Build history of the part. All positions in model axes, mm. Face numbers are marked on the shaded views. A direction names the side the tool comes from. Coordinates: 2 decimals unless noted, no trailing zeros. Order: outer loops, then holes, each group sorted by start corner. A loop starts at its lowest first (then second) coordinate and runs counter-clockwise, first axis right, second up. Notation, with made-up numbers: (-23, -3) - (26, -3) arc R19 cw to (26, 16) - close; hole circle Ø1 at (-28, 7). An arc over 180 degrees is marked (long way). Write each question's results on one line, items separated by ' | '.
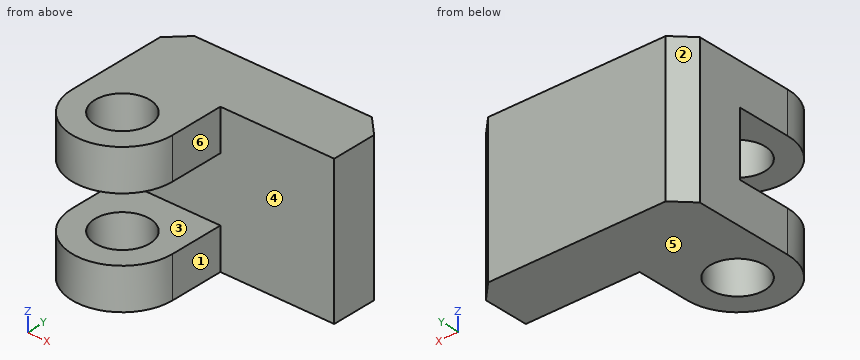
Autodesk Inventor part; units mm, degrees
ref_plane "YZ Plane" through (0, 0, 0) normal (1, 0, 0) x (0, 1, 0)
ref_plane "XZ Plane" through (0, 0, 0) normal (0, 1, 0) x (-1, 0, 0)
ref_plane "XY Plane" through (0, 0, 0) normal (0, 0, 1) x (1, 0, 0)
sketch "스케치1" plane through (0, 0, 0) normal (0, 0, 1) x (1, 0, 0)
  line L0 (0, 0) -> (23.5, 0)
  line L1 (23.5, 0) -> (23.5, -7)
  line L2 (23.5, -7) -> (11, -7)
  line L3 (0, -7) -> (0, 0)
  circle A0 centre (5.5, -13) radius 3
  arc A1 (0, -13) -> (11, -13) centre (5.5, -13) ccw
  line L4 (11, -13) -> (11, -7)
  line L5 (0, -13) -> (0, -7)
  dimension "d0" = 23.5
  dimension "d1" = 7
  dimension "d2" = 6
  dimension "d3" = 6
  dimension "d4" = 5.5
  dimension "d5" = 11
  dimension "d6" = 23.5
extrude "돌출1" add sketch "스케치1" along normal mid plane 16
ref_plane "작업 평면1" through (0, 0, 0) normal (0, 0, 1) x (1, 0, 0)
sketch "스케치2" plane through (0, 0, 0) normal (0, 0, 1) x (1, 0, 0)
  line L0 (-2.9119, -7) -> (15.7404, -7)
  line L1 (15.7404, -7) -> (15.7404, -20.77)
  line L2 (15.7404, -20.77) -> (-2.9119, -20.77)
  line L3 (-2.9119, -20.77) -> (-2.9119, -7)
  line L4 (0, 0) -> (23.5, 0)
  dimension "d9" = 7
extrude "돌출2" cut sketch "스케치2" along normal mid plane 7
chamfer "모따기1" distance 2 angle 45 2 edges at (23.5, 0, 0) (0, 0, 0)
properties part number "2번부품"
1. Two-plate mould, pull along Z, no slides. Class the marked faces 4, 5 and 6: +Z half, -Z half, draft (parallel to the pull), parting line (faces both ways), or undercut.
Solved:
face 4: undercut | face 5: -Z half | face 6: draft
2. Drop flat-ended pins along their axis: pin 1 Ø5 at (y, z) = (-11, -5.5) entering from +X; pin 2 Ø4 at (y, z) = (-15.5, 2.5) entering from +X; pin 3 Ø5 at (x, z) = (14, 2.5) entering from -Y. Give the stop position or say it passes through.
Solved:
pin 1: stops at x = 11 | pin 2: stops at x = 10.95 | pin 3: stops at y = -7
3. Band-saw the part on C-C on z = -6. Give the cut face in (x, y).
Solved:
outline: (0, -13) arc R5.5 ccw to (11, -13) - (11, -7) - (23.5, -7) - (23.5, -2) - (21.5, 0) - (2, 0) - (0, -2) - close; hole circle Ø6 at (5.5, -13)
4. Band-saw the part on A-A on x = 5.5. Give the cut face in (y, z), then the cut area to 4 significant figures.
Solved:
outline: (-18.5, -8) - (-16, -8) - (-16, -3.5) - (-18.5, -3.5) - close; (-18.5, 3.5) - (-16, 3.5) - (-16, 8) - (-18.5, 8) - close; (-10, -8) - (0, -8) - (0, 8) - (-10, 8) - (-10, 3.5) - (-7, 3.5) - (-7, -3.5) - (-10, -3.5) - close | area: 161.5 mm2
5. Probe line 1 (Y direction, x = 5.5, z = 5); line 2 (X direction, y = -13, z = 5.95); line 3 (Z direction, x = 5, y = -8). List the from-to ranges inside material, lowest first.
Solved:
line 1: y = -18.5 to -16, -10 to 0 | line 2: x = 0 to 2.5, 8.5 to 11 | line 3: z = -8 to -3.5, 3.5 to 8
6. Band-saw the part on D-D on y = -14.75. Give the cut face in (x, z).
Solved:
outline: (0.29, -8) - (3.06, -8) - (3.06, -3.5) - (0.29, -3.5) - close; (0.29, 3.5) - (3.06, 3.5) - (3.06, 8) - (0.29, 8) - close; (7.94, -8) - (10.71, -8) - (10.71, -3.5) - (7.94, -3.5) - close; (7.94, 3.5) - (10.71, 3.5) - (10.71, 8) - (7.94, 8) - close
7. Tool access for the marked faces 1, 2 and 3: list every direction of +Z, -Z, +X, -X, +Y, -Y with a clear straight run to the whole face (end or side of a thin tool).
Solved:
face 1: +Z, -Z, +X, -Y | face 2: +Z, -Z, -X, +Y | face 3: +X, -X, -Y
8. Band-saw the part on B-B on y = -9. Give the cut face in (x, z).
Solved:
outline: (0, -8) - (11, -8) - (11, -3.5) - (0, -3.5) - close; (0, 3.5) - (11, 3.5) - (11, 8) - (0, 8) - close
